from build123d import *

# Parameters (mm, degrees)
SKETCH1_W           = 41.760012726
SKETCH1_H           = 40.652739662
SKETCH1_R           = 20
BOSS_EXTRUDE1_DEPTH = 10
BOSS_EXTRUDE2_START = -3
BOSS_EXTRUDE2_DEPTH = 3
SKETCH3_W           = 2
SKETCH3_H           = 2
BOSS_EXTRUDE3_DEPTH = 3


with BuildPart() as part:
    # Sketch1 → Boss-Extrude1 (new body)
    with BuildSketch(Plane.XY):
        Rectangle(SKETCH1_W, SKETCH1_H)
        Circle(SKETCH1_R, mode=Mode.SUBTRACT)
    extrude(amount=BOSS_EXTRUDE1_DEPTH)

    # Sketch2 → Boss-Extrude2 (add)
    with BuildSketch(Plane.XY.offset(10).offset(BOSS_EXTRUDE2_START)):
        with BuildLine():
            Line((-7.096476546, 8.702942047), (5.729829486, 19.161655828))
            ThreePointArc((5.729829486, 19.161655828), (8.229395138, 18.228468275), (10.582504972, 16.970874713))
            Line((10.582504972, 16.970874713), (4.075462496, 10.463832237))
            ThreePointArc((4.075462496, 10.463832237), (1.74837497, -11.092536437), (-7.096476546, 8.702942047))
        make_face()
    extrude(amount=BOSS_EXTRUDE2_DEPTH)

    # Sketch3 → Boss-Extrude3 (add)
    with BuildSketch(Plane.XY.offset(10)):
        with Locations((15.395513793, -16.659790737)):
            Rectangle(SKETCH3_W, SKETCH3_H)
        with Locations((17.287307426, 17.672760389)):
            Rectangle(SKETCH3_W, SKETCH3_H)
        with Locations((-18.796904472, -16.691717232)):
            Rectangle(SKETCH3_W, SKETCH3_H)
        with Locations((-18.236373025, 17.672760389)):
            Rectangle(SKETCH3_W, SKETCH3_H)
    extrude(amount=BOSS_EXTRUDE3_DEPTH)


solid = part.part
Geometry check sheet. Reference: the model listing, model coordinates, mm. A direction names the side the tool comes from. Round coordinates to 2 decimals unless told otherwise and drop trailing zeros. Order: outer loops, then holes, each group sorted by start corner. A loop starts at its lowest first (then second) coordinate and runs counter-clockwise, first axis right, second up. Notation, with made-up numbers: (-33.75, 64) -> (-20.75, 64) arc R34 ccw to (-20.75, 98) -> close; hole circle Ø4 at (24.25, -3.5). An arc over 180 degrees is marked (long way). Use one line per item in the form item = value.
1. Scan lines: line 1 along X through (y, z) = (0, 7.25); line 2 along X through (y, z) = (0, 4.5); line 3 along Y through (x, z) = (-19, 12). Record each from-to range of solid material in increasing order. Write a range as from..to.
Working result:
line_1 = -20.88..-20, -11.23..11.23, 20..20.88
line_2 = -20.88..-20, 20..20.88
line_3 = -17.69..-15.69, 16.67..18.67
2. Set-up check for faces 1 (the face through (-0.77, 13.86, 8.48)), 2 (the face through (-18, 16.673, 11)), 3 (the face through (-19.797, -17, 11)): record each of +Z, -Z, +X, -X, +Y, -Y from which the full face is reachable in a straight line by a thin tool's end or side.
Working result:
face_1 = +Z, -Z
face_2 = +Z, +X, -X
face_3 = +Z, -X, +Y, -Y
3. Mould release check, pull along X, two halves, no side actions. Record for faces 4 (the face through (7.37, 13.76, 8.48)), 5 (the face through (18.287, 18, 11)), 6 (the face through (0, 20.326, 5)), 7 (the face through (14.396, -17, 11)): pulls with the +X half, pulls with the -X half, needs draft (parallel to the pull), parting line crosses it, or undercut.
Working result:
face_4 = undercut
face_5 = pulls with the +X half
face_6 = needs draft
face_7 = undercut
4. Cross-section at A-A, the plane y = 0. Enter the section's corners in (x, z), plus the area to 3 significant figures.
Working result:
outline = (-20.88, 0) -> (-20, 0) -> (-20, 10) -> (-20.88, 10) -> close; (-11.23, 7) -> (11.23, 7) -> (11.23, 10) -> (-11.23, 10) -> close; (20, 0) -> (20.88, 0) -> (20.88, 10) -> (20, 10) -> close
area = 85.0 mm^2
5. Cross-section at D-D, the plane z = 2.75. Enter the section's corners in (x, y), plus the area to 3 significant figures.
Working result:
outline = (-20.88, -20.33) -> (20.88, -20.33) -> (20.88, 20.33) -> (-20.88, 20.33) -> close; hole circle Ø40 at (0, 0)
area = 441 mm^2
6. Cross-section at B-B, the plane z = 8. Enter the section's corners in (x, y), plus the area to 3 significant figures.
Working result:
outline = (-20.88, -20.33) -> (20.88, -20.33) -> (20.88, 20.33) -> (-20.88, 20.33) -> close; hole (-7.1, 8.7) -> (5.73, 19.16) arc R20 ccw (long way) to (10.58, 16.97) -> (4.08, 10.46) arc R11.23 cw (long way) to start
area = 896 mm^2
7. Cross-section at C-C, the plane x = 0. Enter the section's corners in (y, z).
Working result:
outline = (-20.33, 0) -> (-20, 0) -> (-20, 10) -> (-20.33, 10) -> close; (-11.23, 7) -> (14.49, 7) -> (14.49, 10) -> (-11.23, 10) -> close; (20, 0) -> (20.33, 0) -> (20.33, 10) -> (20, 10) -> close
8. Go/stop test with flat-tipped pins: pin 1 (0.6 mm diameter, centred on y = -16.5, z = 12, fed in from +X); pin 2 (1 mm diameter, centred on y = 17.5, z = 11, fed in from +X); pin 3 (0.6 mm diameter, centred on y = -16.5, z = 11, fed in from -X). Record where each tip stops, or that it passes through.
Working result:
pin_1 = 16.4
pin_2 = 18.29
pin_3 = -19.8
